Part model, mm, in its own coordinate system. Round coordinates to 2 decimals unless told otherwise and drop trailing zeros. Loops run counter-clockwise (first coordinate to the right, second up) from the corner with the lowest first, then second, coordinate; pieces in that order, holes last. Notation, with made-up numbers: M 71.25,45.5 L 129.25,45.5 A27 cw 129.25,72.5 Z; hole C 67.25,64 d3. An arc over 180 degrees is marked long. Put each result on its own line as item: value. Start each with the question number.
```python
from build123d import *

# Parameters (mm, degrees)
SKETCH1_W                   = 20
SKETCH1_H                   = 10
BOSS_EXTRUDE1_DEPTH         = 5
TAP_DRILL_FOR_M4X0_7_TAP1_D = 3.8
TAP_DRILL_FOR_M4X0_7_TAP2_D = 3.9
TAP_DRILL_FOR_M4X0_7_TAP3_D = 4


with BuildPart() as part:
    # Sketch1 → Boss-Extrude1 (new body)
    with BuildSketch(Plane(origin=(0, 0, 0), x_dir=(1, 0, 0), z_dir=(0, 1, 0))):
        with Locations((10, 5)):
            Rectangle(SKETCH1_W, SKETCH1_H)
    extrude(amount=BOSS_EXTRUDE1_DEPTH)

    # Tap Drill for M4x0.7 Tap1 (through all)
    with Locations(Plane(origin=(4, 5, -5), x_dir=(0, 0, 1), z_dir=(0, 1, 0))):
        with Locations((0, 0)):
            Hole(TAP_DRILL_FOR_M4X0_7_TAP1_D / 2)

    # Tap Drill for M4x0.7 Tap2 (through all)
    with Locations(Plane(origin=(10, 5, -5), x_dir=(0, 0, 1), z_dir=(0, 1, 0))):
        with Locations((0, 0)):
            Hole(TAP_DRILL_FOR_M4X0_7_TAP2_D / 2)

    # Tap Drill for M4x0.7 Tap3 (through all)
    with Locations(Plane(origin=(16, 5, -5), x_dir=(0, 0, 1), z_dir=(0, 1, 0))):
        with Locations((0, 0)):
            Hole(TAP_DRILL_FOR_M4X0_7_TAP3_D / 2)


solid = part.part
```
1. Cut at D-D, the plane x = 16. Give the cut face in (y, z), and give its area (3 significant figures).
2. Cut at B-B, the plane z = -5. Give the cut face in (x, y).
3. Wall check: L1, parallel to X at y = 1, z = -5; L2, parallel to X at y = 2.45, z = -6.5; L3, parallel to Z at x = 4.75, y = 1.95. Give the ranges that are in metal, low to high.
4. Mould opens along Z. For faces 1 (the flat face through (10, 2, -10)), 2 (the cylindrical face through (8.813, 2.465, -3.453)), 3 (the flat face through (0, 2, -5)) say: released by +Z, released by -Z, zero draft, split by the parting line, or undercut.
5. Cut at A-A, the plane x = 10. Give the cut face in (y, z), and give its area (3 significant figures).
6. Cut at C-C, the plane y = 2.35. Give the cut face in (x, z), and give its area (3 significant figures).
Results list:
1. outline: M 0,-10 L 5,-10 L 5,-7 L 0,-7 Z; M 0,-3 L 5,-3 L 5,0 L 0,0 Z
1. area: 30.0 mm^2
2. outline: M 0,0 L 2.1,0 L 2.1,5 L 0,5 Z; M 5.9,0 L 8.05,0 L 8.05,5 L 5.9,5 Z; M 11.95,0 L 14,0 L 14,5 L 11.95,5 Z; M 18,0 L 20,0 L 20,5 L 18,5 Z
3. L1: x = 0 to 2.1, 5.9 to 8.05, 11.95 to 14, 18 to 20
3. L2: x = 0 to 2.83, 5.17 to 8.75, 11.25 to 14.68, 17.32 to 20
3. L3: z = -10 to -6.75, -3.25 to 0
4. face 1: released by -Z
4. face 2: undercut
4. face 3: zero draft
5. outline: M 0,-10 L 5,-10 L 5,-6.95 L 0,-6.95 Z; M 0,-3.05 L 5,-3.05 L 5,0 L 0,0 Z
5. area: 30.5 mm^2
6. outline: M 0,-10 L 20,-10 L 20,0 L 0,0 Z; hole C 4,-5 d3.8; hole C 10,-5 d3.9; hole C 16,-5 d4
6. area: 164 mm^2
